Read the model definition and answer for the solid it produces. Units are mm, in the model's axes. A direction names the side the tool comes from. Coordinates: 2 decimals unless noted, no trailing zeros. Order: outer loops, then holes, each group sorted by start corner. A loop starts at its lowest first (then second) coordinate and runs counter-clockwise, first axis right, second up. Notation, with made-up numbers: (83, 35.25) - (142, 35.25) arc R19 ccw to (142, 65.25) - close; hole circle Ø2 at (10, 89.5). An arc over 180 degrees is marked (long way). Use one line per item in the form item = value.
```python
from build123d import *

# Parameters (mm, degrees)
F0_W     = 17.78
F0_H     = 17.78
F0_R     = 6.35
F1_DEPTH = 25.4
F2_W     = 17.78
F2_H     = 17.78
F3_DEPTH = 17.78
F5_D     = 12.7
F5_DEPTH = 25.4


with BuildPart() as f1:
    # F0 (on Top) → F1 (new body)
    with BuildSketch(Plane.XY):
        with Locations((-39.151133, -30.113884)):
            Rectangle(F0_W, F0_H)
        with Locations((-39.151133, -30.113884)):
            Circle(F0_R, mode=Mode.SUBTRACT)
    extrude(amount=F1_DEPTH)

    # F2 (on face) → F3 (join)
    with BuildSketch(Plane(origin=(0, -21.223884, 0), x_dir=(-1, 0, 0), z_dir=(0, 1, 0))):
        with Locations((39.151133, 12.7)):
            Rectangle(F2_W, F2_H)
    extrude(amount=F3_DEPTH)

    # F5
    with Locations(Plane.YZ.offset(-30.261133)):
        with Locations((-12.333884, 12.7)):
            Hole(F5_D / 2, depth=F5_DEPTH)


solid = f1.part
```
(1) Section D-D, the plane z = 16 is taken. Write down the section's boundary in (x, y).
Answer list:
outline = (-48.04, -39) - (-30.26, -39) - (-30.26, -17.76) - (-48.04, -17.76) - close; (-48.04, -6.91) - (-30.26, -6.91) - (-30.26, -3.44) - (-48.04, -3.44) - close; hole circle Ø12.7 at (-39.15, -30.11)
(2) Given pin 1 Ø9 at (x, y) = (-43, -12) entering from -Z; pin 2 Ø5.5 at (x, y) = (-42, -15.5) entering from +Z, each flat-ended and moving along its own axis, determine where each tip first touches the part or whether it passes through.
Answer list:
pin_1 = 3.81
pin_2 = 21.59
(3) The mould has two halves that part along Y. Classify faces 1 (the flat face through (-39, -12, 21.59)), 2 (the flat face through (-39, -39.004, 13)), 3 (the cylindrical face through (-39.276, -15.748, 18.054)): +Y half, -Y half, draft (parallel to the pull), parting line (faces both ways), or undercut.
Answer list:
face_1 = draft
face_2 = -Y half
face_3 = undercut
(4) Section A-A, the plane z = 10.5 is taken. Write down the section's boundary in (x, y).
Answer list:
outline = (-48.04, -39) - (-30.26, -39) - (-30.26, -18.29) - (-48.04, -18.29) - close; (-48.04, -6.38) - (-30.26, -6.38) - (-30.26, -3.44) - (-48.04, -3.44) - close; hole circle Ø12.7 at (-39.15, -30.11)
(5) Section C-C, the plane y = -13 is taken. Write down the section's boundary in (x, z), then the cut area to 3 significant figures.
Answer list:
outline = (-48.04, 3.81) - (-30.26, 3.81) - (-30.26, 6.39) - (-48.04, 6.39) - close; (-48.04, 19.01) - (-30.26, 19.01) - (-30.26, 21.59) - (-48.04, 21.59) - close
area = 91.6 mm2
(6) Section B-B, the plane x = -45 is taken. Write down the section's boundary in (y, z), then the cut area to 3 significant figures.
Answer list:
outline = (-39, 0) - (-32.59, 0) - (-32.59, 25.4) - (-39, 25.4) - close; (-27.64, 0) - (-21.22, 0) - (-21.22, 3.81) - (-3.44, 3.81) - (-3.44, 21.59) - (-21.22, 21.59) - (-21.22, 25.4) - (-27.64, 25.4) - close; hole circle Ø12.7 at (-12.33, 12.7)
area = 515 mm2
(7) Which of the six approach directions +Z, -Z, +X, -X, +Y, -Y give full straight-line access (tool end or side, diameter ignored) to faces 4 (the flat face through (-39, -12, 3.81)), 5 (the flat face through (-48.041, -25, 13)), 6 (the flat face through (-39, -21.224, 23))?
Answer list:
face_4 = -Z, +X, -X, +Y
face_5 = +Z, -Z, -X, +Y, -Y
face_6 = +Z, +X, -X, +Y
(8) Straight lines are drawn through the part: L1, parallel to Y at x = -39, z = 11.75; L2, parallel to Y at x = -39, z = 7.25; L3, parallel to Y at x = -39.5, z = 24.25. For each, find the intervals that lie inside material, in ascending order.
Answer list:
L1 = -39 to -36.46, -23.77 to -18.61, -6.06 to -3.44
L2 = -39 to -36.46, -23.77 to -15.59, -9.08 to -3.44
L3 = -39 to -36.45, -23.77 to -21.22
